The listing builds one solid part. Answer for the finished solid, in the listing's coordinates (mm). Face numbers are marked on the shaded views. A direction names the side the tool comes from. Coordinates: 2 decimals unless noted, no trailing zeros. Loops run counter-clockwise (first coordinate to the right, second up) from the corner with the lowest first, then second, coordinate; pieces in that order, holes last. Notation, with made-up numbers: (-4, -25.5) - (23, -25.5) arc R15 cw to (23, 2.5) - close; hole circle Ø2 at (-29, 55). An arc over 180 degrees is marked (long way). Return JSON: item names as keys, results as strings. Group by question number.
1. Section B-B (z = 5) is taken. Write down the section's boundary in (x, y) (3 decimals), and give its area (3 significant figures).
2. Which of the six approach directions +Z, -Z, +X, -X, +Y, -Y give full straight-line access (tool end or side, diameter ignored) to the marked faces 1 and 2?
3. Find the intervals of material crossed by line 1 along Z through (x, y) = (12.25, 2.5); line 2 along Z through (x, y) = (12.75, 2.5); line 3 along X through (y, z) = (9, -20) (3 decimals), in increasing order.
4. Section A-A (x = 13.75) is taken. Write down the section's boundary in (y, z) (3 decimals).
5. Each of these flat-tipped pins is pushed along its axis until it touches: P1, Ø5, axis at y = 8.5, z = -20, coming from the +X side (3 decimals); P2, Ø12, axis at x = 9.5, z = 61, coming from the +Y side (3 decimals); P3, Ø4, axis at x = 14.29, z = 74.39, coming from the +Y side. Where does it stop, or does it pass through?
6. Section C-C (y = 6.75) is taken. Write down the section's boundary in (x, z) (3 decimals), and give its area (3 significant figures).
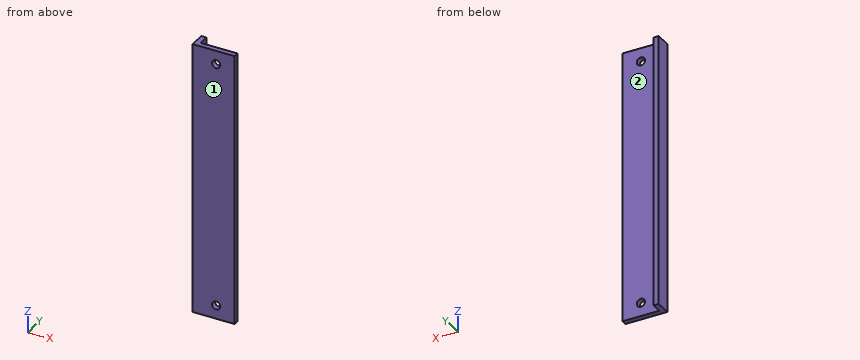
```python
from build123d import *

# Parameters (mm, degrees)
BOSS_EXTRUDE1_DEPTH = 82.55
SKETCH2_R           = 2.4892
CUT_EXTRUDE4_DEPTH  = 10.525


with BuildPart() as part:
    # Sketch1 → Boss-Extrude1 (new body, symmetric)
    with BuildSketch(Plane.XY):
        Polygon((0, 9.525), (0, 0), (25.4, 0), (25.4, 3.175), (3.175, 3.175), (3.175, 9.525), align=None)
    extrude(amount=BOSS_EXTRUDE1_DEPTH, both=True)

    # Sketch2 → Cut-Extrude4 (cut, through all)
    with BuildSketch(Plane(origin=(0, 0, 0), x_dir=(1, 0, 0), z_dir=(0, 1, 0))):
        with Locations((14.2875, -74.3926249)):
            Circle(SKETCH2_R)
        with Locations((14.2875, 74.3926249)):
            Circle(SKETCH2_R)
    extrude(amount=CUT_EXTRUDE4_DEPTH, mode=Mode.SUBTRACT)


solid = part.part
```
The answers:
{
 "1": {"outline": "(0, 0) - (25.4, 0) - (25.4, 3.175) - (3.175, 3.175) - (3.175, 9.525) - (0, 9.525) - close", "area": "101 mm2"},
 "2": {"face 1": "+Z, -Z, +X, -X, -Y", "face 2": "+Z, -Z, +X, +Y"},
 "3": {"line 1": "z = -82.55 to -75.82, -72.96 to 72.96, 75.82 to 82.55", "line 2": "z = -82.55 to -76.35, -72.44 to 72.44, 76.35 to 82.55", "line 3": "x = 0 to 3.175"},
 "4": {"outline": "(0, -82.55) - (3.175, -82.55) - (3.175, -76.823) - (0, -76.823) - close; (0, -71.962) - (3.175, -71.962) - (3.175, 71.962) - (0, 71.962) - close; (0, 76.823) - (3.175, 76.823) - (3.175, 82.55) - (0, 82.55) - close"},
 "5": {"P1": "stops at x = 3.175", "P2": "stops at y = 3.175", "P3": "passes through"},
 "6": {"outline": "(0, -82.55) - (3.175, -82.55) - (3.175, 82.55) - (0, 82.55) - close", "area": "524 mm2"}
}
